Autodesk Inventor part; units mm, degrees
ref_plane "MiddlePlane" through (7.8315, 65.9547, 5) normal (1, 0, 0) x (0, 0, -1)
ref_plane "YZ Plane" through (0, 0, 0) normal (1, 0, 0) x (0, 1, 0)
ref_plane "XZ Plane" through (0, 0, 0) normal (0, 1, 0) x (-1, 0, 0)
sketch "Body" plane through (0, 0, 0) normal (0, 0, 1) x (1, 0, 0)
  line L0 (-42.1685, 50.6373) -> (57.8315, 50.6373) construction
  line L1 (-42.1685, 50.6373) -> (-42.1685, 45.6373) construction
  line L2 (-42.1685, 45.6373) -> (-31.6685, 45.6373) construction
  line L3 (-31.6685, 45.6373) -> (-31.6685, 18.1373) construction
  line L4 (-31.6685, 18.1373) -> (-42.1685, 18.1373) construction
  line L5 (-42.1685, 18.1373) -> (-42.1685, 13.1373) construction
  line L6 (-42.1685, 13.1373) -> (57.8315, 13.1373) construction
  line L7 (57.8315, 18.1373) -> (57.8315, 13.1373) construction
  line L8 (47.3315, 18.1373) -> (57.8315, 18.1373) construction
  line L9 (47.3315, 45.6373) -> (47.3315, 18.1373) construction
  line L10 (57.8315, 45.6373) -> (47.3315, 45.6373) construction
  line L11 (57.8315, 50.6373) -> (57.8315, 45.6373) construction
  circle A0 centre (40.0815, 25.3873) radius 3.25 construction
  arc A1 (28.5815, 34.3873) -> (28.5815, 37.8873) centre (28.5815, 36.1373) ccw construction
  line L12 (15.0815, 34.3873) -> (28.5815, 34.3873) construction
  arc A2 (15.0815, 37.8873) -> (15.0815, 34.3873) centre (15.0815, 36.1373) ccw construction
  line L13 (28.5815, 37.8873) -> (15.0815, 37.8873) construction
  line L14 (29.0815, 28.6373) -> (16.5815, 28.6373)
  arc A3 (29.0815, 22.1373) -> (29.0815, 28.6373) centre (29.0815, 25.3873) ccw
  line L15 (16.5815, 22.1373) -> (29.0815, 22.1373)
  arc A4 (16.5815, 28.6373) -> (16.5815, 22.1373) centre (16.5815, 25.3873) ccw
  line L16 (-13.4185, 28.6373) -> (-0.9185, 28.6373)
  arc A5 (-0.9185, 22.1373) -> (-0.9185, 28.6373) centre (-0.9185, 25.3873) ccw
  line L17 (-0.9185, 22.1373) -> (-13.4185, 22.1373)
  arc A6 (-13.4185, 28.6373) -> (-13.4185, 22.1373) centre (-13.4185, 25.3873) ccw
  arc A7 (-12.9185, 37.8873) -> (-12.9185, 34.3873) centre (-12.9185, 36.1373) ccw construction
  line L18 (-12.9185, 37.8873) -> (0.5815, 37.8873) construction
  arc A8 (0.5815, 34.3873) -> (0.5815, 37.8873) centre (0.5815, 36.1373) ccw construction
  line L19 (0.5815, 34.3873) -> (-12.9185, 34.3873) construction
  circle A9 centre (-24.4185, 25.3873) radius 3.25 construction
  line L20 (6.8315, 42.6373) -> (8.8315, 42.6373) construction
  arc A10 (8.8315, 39.1373) -> (8.8315, 42.6373) centre (8.8315, 40.8873) ccw construction
  line L21 (6.8315, 39.1373) -> (8.8315, 39.1373) construction
  arc A11 (6.8315, 42.6373) -> (6.8315, 39.1373) centre (6.8315, 40.8873) ccw construction
  circle A12 centre (40.0815, 25.3873) radius 7.25
  circle A13 centre (-24.4185, 25.3873) radius 7.25
  line L22 (40.0815, 25.3873) -> (40.0815, 18.1373) construction
  line L23 (-24.4185, 18.1373) -> (40.0815, 18.1373)
  line L24 (-24.4185, 25.3873) -> (-24.4185, 18.1373) construction
  line L25 (40.0815, 25.3873) -> (40.0815, 32.6373) construction
  line L26 (-24.4185, 25.3873) -> (-24.4185, 32.6373) construction
  line L27 (40.0815, 32.6373) -> (24.0815, 32.6373)
  line L28 (24.0815, 32.6373) -> (15.3024, 50.6373)
  line L29 (15.3024, 50.6373) -> (0.3607, 50.6373)
  line L30 (0.3607, 50.6373) -> (-8.4185, 32.6373)
  line L31 (-8.4185, 32.6373) -> (-24.4185, 32.6373)
  line L32 (8.8315, 40.8873) -> (6.8315, 40.8873) construction
  circle A14 centre (7.8315, 40.8873) radius 1.5
  circle A15 centre (0.5815, 36.1373) radius 1.5
  circle A16 centre (15.0815, 36.1373) radius 1.5
  circle A17 centre (40.0815, 25.3873) radius 3
  circle A18 centre (-24.4185, 25.3873) radius 3
  dimension "d2" = 16
  dimension "d3" = 16
  dimension "d4" = 116
  dimension "d8" = 3
  dimension "d9" = 3
  dimension "d10" = 3
  dimension "d11" = 6
  dimension "d12" = 6
extrude "BodyFeature" add sketch "Body" along normal blind 5
fillet "BodyFilletsFeature" radius 2 4 edges at (24.0815, 32.6373, 2.5) (-8.4185, 32.6373, 2.5) (0.3607, 50.6373, 2.5) (15.3024, 50.6373, 2.5)
ref_plane "MiddlePlane" through (7.8315, 65.9547, 5) normal (1, 0, 0) x (0, 0, -1)
sketch "PelvisSpineBase" plane through (7.8315, 65.9547, 5) normal (1, 0, 0) x (0, 0, -1)
  arc A0 (0, -66.3174) -> (12.5911, -56.659) centre (10, -66.3174) ccw
  circle A1 centre (10, -66.3174) radius 6
  line L0 (5, -33.3174) -> (5, -47.8174) construction
  line L1 (5, -47.8174) -> (0, -47.8174)
  line L2 (0, -47.8174) -> (0, -66.3174)
  line L3 (5, -47.8174) -> (5, -52.8174)
  line L4 (5, -52.8174) -> (10, -52.8174)
  line L5 (10, -52.8174) -> (12.5911, -56.659)
  dimension "d16" = 12
  dimension "d17" = 4
  dimension "d22" = 5
  dimension "d23" = 5
  dimension "d29" = 18.5
  dimension "d30" = 34
extrude "PelvisSpineBaseFeature" add sketch "PelvisSpineBase" along normal mid plane 15
sketch "AngleReinforce" plane through (0, 0, 5) normal (0, 0, 1) x (1, 0, 0)
  line L0 (15.3315, 18.1373) -> (15.3315, 13.1373)
  line L1 (15.3315, 13.1373) -> (15.3315, 18.1373)
  line L2 (15.3315, 13.1373) -> (22.3315, 18.1373)
  line L3 (15.3315, 18.1373) -> (40.0815, 18.1373) construction
  line L4 (15.3315, 18.1373) -> (22.3315, 18.1373)
  line L5 (0.3315, 18.1373) -> (0.3315, 13.1373)
  line L6 (0.3315, 18.1373) -> (0.3315, 13.1373)
  line L7 (0.3315, 13.1373) -> (-6.6685, 18.1373)
  line L8 (-24.4185, 18.1373) -> (0.3315, 18.1373) construction
  line L9 (0.3315, 18.1373) -> (-6.6685, 18.1373)
  dimension "d33" = 7
  dimension "d34" = 7
extrude "AngleReinforceFeature" add sketch "AngleReinforce" against normal blind 2
sketch "RightLip" plane through (15.3315, 65.9547, 5) normal (1, 0, 0) x (0, 0, -1)
  arc A0 (0, -66.3174) -> (12.5911, -56.659) centre (10, -66.3174) ccw
  circle A1 centre (10, -66.3174) radius 10
  circle A2 centre (10, -66.3174) radius 9
  dimension "d37" = 1
extrude "RightLipFeature" cut sketch "RightLip" against normal blind 1
sketch "LeftLip" plane through (0.3315, 65.9547, 5) normal (-1, 0, 0) x (0, 0, 1)
  arc A0 (-12.5911, -56.659) -> (0, -66.3174) centre (-10, -66.3174) ccw
  circle A1 centre (-10, -66.3174) radius 9
  circle A2 centre (-10, -66.3174) radius 10
  dimension "d40" = 1
extrude "LeftLipFeature" cut sketch "LeftLip" against normal blind 1
fillet "SharpEdgesFilletFeature" radius 1 4 edges at (0.8315, -0.3627, 5) (0.8315, 9.2958, -7.5911) (14.8315, 9.2958, -7.5911) (14.8315, -0.3627, 5)
equation "\"d3\" = d2"
properties part number "PelvisSpineLink"
Model file for the job. Use its own axes, mm. A direction names the side the tool comes from. Give positions to 0.01 mm unless a question says otherwise; leave off trailing zeros. Loops run counter-clockwise (first coordinate to the right, second up) from the corner with the lowest first, then second, coordinate; pieces in that order, holes last. Notation, with made-up numbers: (-8.5, 7) - (47.5, 7) arc R12 ccw to (47.5, 26) - close; hole circle Ø1 at (31, -32.5). An arc over 180 degrees is marked (long way). Use one line per item in the form item = value.
(1) Cut at B-B (y = 2). Give the cut face in (x, z), then the cut area to 3 significant figures.
Determined:
outline = (0.33, -13.68) - (1.33, -13.68) - (1.33, -14.72) - (14.33, -14.72) - (14.33, -13.68) - (15.33, -13.68) - (15.33, -10.52) - (0.33, -10.52) - close; (0.33, 0.52) - (15.33, 0.52) - (15.33, 3.68) - (14.33, 3.68) - (14.33, 5) - (1.33, 5) - (1.33, 3.68) - (0.33, 3.68) - close
area = 126 mm^2
(2) Drop flat-ended pins along their axis: P1, Ø9, axis at y = -3.5, z = -2, coming from the -X side; P2, Ø4, axis at x = -9.5, z = 3.5, coming from the +Y side; P3, Ø1.5, axis at x = 5.5, z = -2.5, coming from the +Y side. Give the stop position or say it passes through.
Determined:
P1 = 0.33
P2 = 34.52
P3 = 13.14
(3) Cut at A-A (x = -5.5). Give the cut face in (y, z).
Determined:
outline = (17.3, 3) - (18.14, 3) - (18.14, 0) - (22.14, 0) - (22.14, 5) - (17.3, 5) - close; (28.64, 0) - (38.62, 0) - (38.62, 5) - (28.64, 5) - close
(4) Pull direction Y, two halves, no side cores. Call faces 4 (the face through (30, 18.137, 2)), 5 (the face through (2.33, 25.46, 2.46)), 6 (the face through (-8.622, 32.933, 2.535)): pulls with the +Y half, pulls with the -Y half, needs draft (parallel to the pull), parting line crosses it, or undercut.
Determined:
face_4 = pulls with the -Y half
face_5 = undercut
face_6 = pulls with the +Y half
(5) 3-axis set-ups, long thin cutter, end or side, ignore diameter. For faces 1 (the face through (-12, 18.137, 2)), 2 (the face through (-7, 28.637, 2)), 3 (the face through (14.84, 8.64, -0.65)): which of +Z, -Z, +X, -X, +Y, -Y reach the whole face in a straight line?
Determined:
face_1 = -Z, -X, -Y
face_2 = +Z, -Z
face_3 = +X
(6) Drill centre lines: L1, parallel to X at y = 28, z = 3.75; L2, parallel to Y at x = 28.5, z = 2; L3, parallel to X at y = 13.5, z = 3.25. Where is each one in solid material? Low to high.
Determined:
L1 = -31.18 to -25.89, -22.94 to -15.35, 1.01 to 14.65, 31.01 to 38.61, 41.56 to 46.84
L2 = 18.14 to 22.14, 28.64 to 32.64
L3 = -0.18 to 15.84
(7) Cut at D-D (y = 14). Give the cut face in (x, z).
Determined:
outline = (-0.88, 3) - (0.33, 3) - (0.33, 0) - (15.33, 0) - (15.33, 3) - (16.54, 3) - (16.54, 5) - (-0.88, 5) - close
(8) Cut at C-C (z = -2). Give the cut face in (x, y).
Determined:
outline = (0.33, -8.85) - (1.33, -8.85) - (1.33, -9.9) - (14.33, -9.9) - (14.33, -8.85) - (15.33, -8.85) - (15.33, -5.56) - (0.33, -5.56) - close; (0.33, 4.83) - (15.33, 4.83) - (15.33, 8.12) - (14.33, 8.12) - (14.33, 9.18) - (15.33, 9.18) - (15.33, 13.14) - (0.33, 13.14) - (0.33, 9.18) - (1.33, 9.18) - (1.33, 8.12) - (0.33, 8.12) - close
